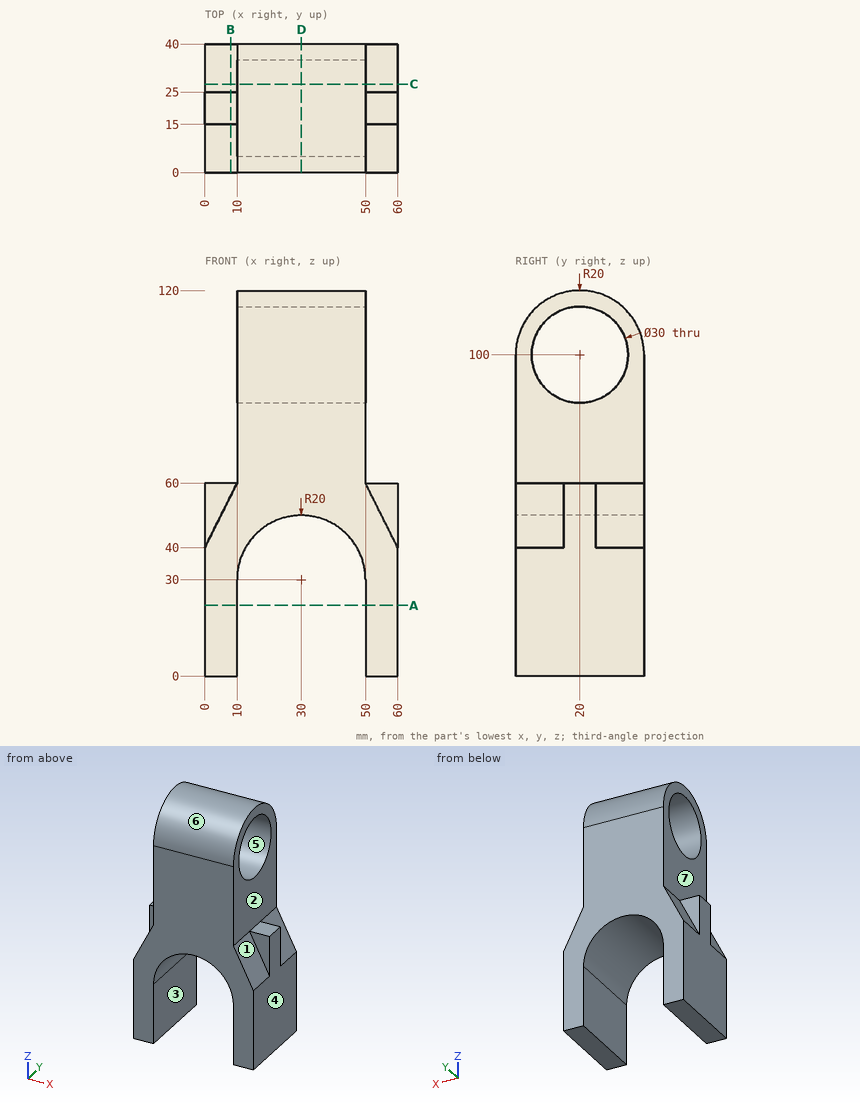
Design review of the part shown in the three views and the two pictorial views. Dimensions are in mm from the part's minimum x, y and z. A direction names the side the tool comes from. Coordinates: 2 decimals unless noted, no trailing zeros. Write each loop counter-clockwise with the first axis right and the second up, starting at its lowest first coordinate (ties: lowest second). Pieces come first, ordered by that corner, then holes.
(1) Add section D-D on x = 30. Give the boundary of the cut face in (y, z), then the cut area to 3 significant figures.
(2) The part is to be moulded in two halves that separate along Z. For the marked faces 5, 6 and 7, say which applies: +Z half, -Z half, draft (parallel to the pull), parting line (faces both ways), or undercut.
(3) Add section C-C on y = 27.5. Give the boundary of the cut face in (x, z).
(4) Add section B-B on x = 8. Give the boundary of the cut face in (y, z), then the cut area to 3 significant figures.
(5) Add section A-A on z = 22. Give the boundary of the cut face in (x, y), then the cut area to 3 significant figures.
(6) Wall thickness on probe 1 along Y at (x, z) = (19.5, 100); probe 2 along X at (y, z) = (5, 28.5); probe 3 along Z at (x, y) = (30, 20): over which ranges is each line inside the solid? List them lowest first.
(7) For pin 1 Ø8 at (x, y) = (30.5, 11) entering from -Z; pin 2 Ø3 at (x, y) = (37.5, 4.5) entering from +Z; pin 3 Ø8 at (x, y) = (2.5, 19.5) entering from +Z, all flat-tipped, find the tip position at first contact; note any pin that passes through.
(8) Tool access review of the marked faces 1, 2, 3 and 4: name each direction out of +Z, -Z, +X, -X, +Y, -Y from which nothing blocks a thin tool from reaching the whole face with its end or side.
Answer sheet:
1. outline: (0, 50) - (40, 50) - (40, 100) arc R20 ccw to (0, 100) - close; hole circle Ø30 at (20, 100)
1. area: 1,920 mm2
2. face 5: undercut
2. face 6: +Z half
2. face 7: draft
3. outline: (0, 0) - (10, 0) - (10, 30) arc R20 cw to (50, 30) - (50, 0) - (60, 0) - (60, 40) - (50, 60) - (50, 87.01) - (10, 87.01) - (10, 60) - (0, 40) - close; (10, 112.99) - (50, 112.99) - (50, 118.54) - (10, 118.54) - close
4. outline: (0, 0) - (40, 0) - (40, 56) - (25, 56) - (25, 60) - (15, 60) - (15, 56) - (0, 56) - close
4. area: 2,280 mm2
5. outline: (0, 0) - (10, 0) - (10, 40) - (0, 40) - close; (50, 0) - (60, 0) - (60, 40) - (50, 40) - close
5. area: 800 mm2
6. probe 1: y = 0 to 5, 35 to 40
6. probe 2: x = 0 to 10, 50 to 60
6. probe 3: z = 50 to 85, 115 to 120
7. pin 1: stops at z = 49.49
7. pin 2: stops at z = 114.28
7. pin 3: stops at z = 60
8. face 1: +Z, +X, -Y
8. face 2: +Z, +X, +Y, -Y
8. face 3: -Z, +Y, -Y
8. face 4: +Z, -Z, +X, +Y, -Y
